Autodesk Inventor part; units mm, degrees
ref_plane "YZ Plane" through (0, 0, 0) normal (1, 0, 0) x (0, 1, 0)
ref_plane "XZ Plane" through (0, 0, 0) normal (0, 1, 0) x (-1, 0, 0)
ref_plane "XY Plane" through (0, 0, 0) normal (0, 0, 1) x (1, 0, 0)
sketch "Boceto1" plane through (0, 0, 0) normal (1, 0, 0) x (0, 1, 0)
  circle A0 centre (0, 0) radius 3.5
  dimension "d0" = 7
extrude "Extrusión1" add sketch "Boceto1" along normal mid plane 38
sketch "Boceto2" plane through (0, 0, 0) normal (1, 0, 0) x (0, 1, 0)
  arc A0 (20.1106, 16.4792) -> (20.1106, -16.4792) centre (26, 0) ccw
  arc A1 (-20.1106, -16.4792) -> (-20.1106, 16.4792) centre (-26, 0) ccw
  arc A2 (-20.1106, -16.4792) -> (20.1106, -16.4792) centre (0, 0) ccw
  arc A3 (20.1106, 16.4792) -> (-20.1106, 16.4792) centre (0, 0) ccw
  dimension "d22" = 35
  dimension "d23" = 35
extrude "Extrusión2" add sketch "Boceto2" along normal mid plane 10
sketch "Boceto3" plane through (0, 0, 0) normal (1, 0, 0) x (0, 1, 0)
  circle A0 centre (0, 0) radius 10
  dimension "d8" = 20
extrude "Extrusión3" add sketch "Boceto3" along normal mid plane 12
sketch "Boceto4" plane through (0, 0, 0) normal (1, 0, 0) x (0, 1, 0)
  circle A0 centre (0, 0) radius 3.5
  circle A1 centre (0, 0) radius 7
  dimension "d11" = 14
extrude "Extrusión4" add sketch "Boceto4" along normal mid plane 20
sketch "Boceto6" plane through (0, 0, 0) normal (0, 1, 0) x (-1, 0, 0)
  line L0 (10, -3.5) -> (10, 3.5)
  line L1 (10, 0) -> (9, 0)
  line L2 (9, 0) -> (9, -10)
  line L3 (9, -10) -> (10, -10)
  line L4 (10, -10) -> (10, 0)
  line L5 (26.6, 0) -> (-26.6, 0)
  point P0 (0, 0)
  dimension "d15" = 1
  dimension "d16" = 10
revolve "Revolución1" add sketch "Boceto6" angle 360 about axis through (-10, 0, 0) along (1, 0, 0)
sketch "Boceto7" plane through (0, 0, 0) normal (0, 1, 0) x (-1, 0, 0)
  line L0 (-10, 7) -> (-10, -7)
  line L1 (-10, 0) -> (-9, 0)
  line L2 (-9, 0) -> (-9, -10)
  line L3 (-9, -10) -> (-10, -10)
  line L4 (-10, -10) -> (-10, 0)
  line L5 (26.6, 0) -> (-26.6, 0)
  point P0 (0, 0)
  dimension "d18" = 1
  dimension "d19" = 10
revolve "Revolución2" add sketch "Boceto7" angle 360 about axis through (-10, 0, 0) along (1, 0, 0)
properties part number "arma" material "Aluminio 6061"
Part model, mm, in its own coordinate system. A direction names the side the tool comes from. Round coordinates to 2 decimals unless told otherwise and drop trailing zeros. Loops run counter-clockwise (first coordinate to the right, second up) from the corner with the lowest first, then second, coordinate; pieces in that order, holes last.
Item 1: Cut at B-B, the plane z = 0. Give the cut face in (x, y).
Item 2: Cut at D-D, the plane y = -16. Give the cut face in (x, z), then the cut area to 3 significant figures.
Item 3: Mould opens along Z. For faces 4 (the face through (19, 0, 0)), 5 (the face through (-0.07, 12.97, 11.68)), 6 (the face through (-0.07, -12.97, -11.68)), 7 (the face through (9.51, -9.76, 2.17)) say: +Z half, -Z half, draft (parallel to the pull), parting line (faces both ways), or undercut.
Item 4: Drop flat-ended pins along their axis: P1, Ø10, axis at x = -6, z = -3, coming from the +Y side; P2, Ø4, axis at y = 11.5, z = -17, coming from the +X side; P3, Ø12, axis at x = 4.5, y = -6.5, coming from the +Z side. Give the stop position or say it passes through.
Item 5: Cut at A-A, the plane y = 13.5. Give the cut face in (x, z), then the cut area to 3 significant figures.
Item 6: Cut at C-C, the plane x = -2.5. Give the cut face in (y, z), then the cut area to 3 significant figures.
Item 7: 3-axis set-ups, long thin cutter, end or side, ignore diameter. For faces 1 (the face through (-6, 2, 7)), 2 (the face through (-0.07, -13.13, 11.86)), 3 (the face through (-10, 0, -4)): which of +Z, -Z, +X, -X, +Y, -Y reach the whole face in a straight line?
Item 8: Drill centre lines: line 1 (X direction, y = 8, z = -2.5); line 2 (X direction, y = 8.5, z = -15.5); line 3 (Y direction, x = 5.5, z = -8). Where is each one in solid material? Low to high.
A:
1. outline: (-19, -3.5) - (-10, -3.5) - (-10, -10) - (-9, -10) - (-9, -7) - (-6, -7) - (-6, -10) - (6, -10) - (6, -7) - (9, -7) - (9, -10) - (10, -10) - (10, -3.5) - (19, -3.5) - (19, 3.5) - (10, 3.5) - (10, 10) - (9, 10) - (9, 7) - (6, 7) - (6, 10) - (-6, 10) - (-6, 7) - (-9, 7) - (-9, 10) - (-10, 10) - (-10, 3.5) - (-19, 3.5) - close
2. outline: (-5, -20.49) - (5, -20.49) - (5, -14.36) - (-5, -14.36) - close; (-5, 14.36) - (5, 14.36) - (5, 20.49) - (-5, 20.49) - close
2. area: 123 mm2
3. face 4: draft
3. face 5: undercut
3. face 6: undercut
3. face 7: parting line
4. P1: stops at y = 10.38
4. P2: stops at x = 5
4. P3: stops at z = 26
5. outline: (-5, -22.22) - (5, -22.22) - (5, -12.25) - (-5, -12.25) - close; (-5, 12.25) - (5, 12.25) - (5, 22.22) - (-5, 22.22) - close
5. area: 199 mm2
6. outline: (-20.11, -16.48) arc R26 ccw to (20.11, -16.48) arc R17.5 cw to (9.03, -4.29) arc R10 ccw to (9.03, 4.29) arc R17.5 cw to (20.11, 16.48) arc R26 ccw to (-20.11, 16.48) arc R17.5 cw to (-9.03, 4.29) arc R10 ccw to (-9.03, -4.29) arc R17.5 cw to start
6. area: 1,320 mm2
7. face 1: none
7. face 2: +X, -X, -Y
7. face 3: -X
8. line 1: x = -10 to -9, -6 to 6, 9 to 10
8. line 2: x = -5 to 5
8. line 3: y = -6 to 6
